For this review, use the dimensioned drawing (mm, ordinates from the lowest corner) and the shaded views. A direction names the side the tool comes from. Give positions to 0.01 mm unless a question says otherwise; leave off trailing zeros. Loops run counter-clockwise (first coordinate to the right, second up) from the corner with the lowest first, then second, coordinate; pieces in that order, holes last. Notation, with made-up numbers: M 75.25,-9.5 L 128.25,-9.5 A9 ccw 128.25,5.5 Z; hole C 84.25,37 d3. An arc over 180 degrees is marked long. Return JSON: item names as keys, results as strings.
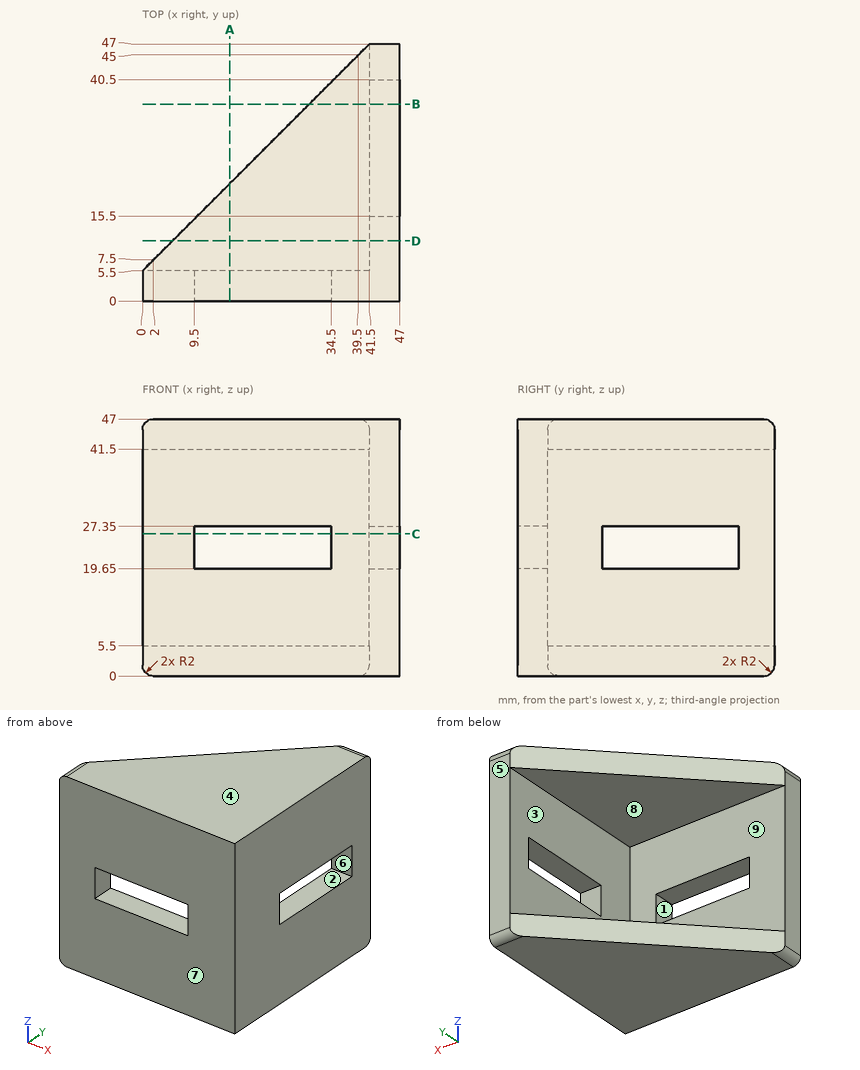
1) Tool access review of the marked faces 1, 2, 3, 4 and 5: name each direction out of +Z, -Z, +X, -X, +Y, -Y from which nothing blocks a thin tool from reaching the whole face with its end or side.
From the geometry:
{"face 1": "+Y, -Y", "face 2": "+X, -X", "face 3": "-X, +Y", "face 4": "+Z, +X, -X, +Y, -Y", "face 5": "+Z, -Z, +X, -X, +Y"}
2) Consider section A-A on x = 16. Write out the cut boundary in (y, z), then the cut area to 3 significant figures.
From the geometry:
{"outline": "M 0,0 L 21.5,0 L 21.5,5.5 L 5.5,5.5 L 5.5,19.65 L 0,19.65 Z; M 0,27.35 L 5.5,27.35 L 5.5,41.5 L 21.5,41.5 L 21.5,47 L 0,47 Z", "area": "392 mm²"}
3) Consider section C-C on z = 26. Write out the cut boundary in (x, y).
From the geometry:
{"outline": "M 0,0 L 9.5,0 L 9.5,5.5 L 0,5.5 Z; M 34.5,0 L 47,0 L 47,15.5 L 41.5,15.5 L 41.5,5.5 L 34.5,5.5 Z; M 41.5,40.5 L 47,40.5 L 47,47 L 41.5,47 Z"}
4) Consider section B-B on y = 36. Write out the cut boundary in (x, z), then the cut area to 3 significant figures.
From the geometry:
{"outline": "M 30.5,0 L 47,0 L 47,19.65 L 41.5,19.65 L 41.5,5.5 L 30.5,5.5 Z; M 30.5,41.5 L 41.5,41.5 L 41.5,27.35 L 47,27.35 L 47,47 L 30.5,47 Z", "area": "337 mm²"}
5) Wall thickness on L1, parallel to Z at x = 9.5, y = 10; L2, parallel to Y at x = 7.5, z = 15; L3, parallel to X at y = 28, z = 16: over which ranges is each line inside the solid? List them lowest first. Write a range as from..to.
From the geometry:
{"L1": "0..5.5, 41.5..47", "L2": "0..5.5", "L3": "41.5..47"}
6) The part is to be moulded in two halves that separate along Y. For the marked faces 6, 7, 8 and 9, say which applies: released by +Y, released by -Y, zero draft, split by the parting line, or undercut.
From the geometry:
{"face 6": "undercut", "face 7": "released by -Y", "face 8": "zero draft", "face 9": "released by +Y"}
7) Insertion check: pin 1 (1 mm diameter, centred on y = 33.5, z = 14, fed in from -X); pin 2 (3 mm diameter, centred on x = 26.5, z = 8, fed in from +Y); pin 3 (12 mm diameter, centred on x = 26.5, y = 41.5, fed in from -Z). Each pin has a flat end and moves straight along its axis. Give the tip position at first contact, or say it passes through.
From the geometry:
{"pin 1": "x = 41.5", "pin 2": "y = 5.5", "pin 3": "through"}
8) Consider section D-D on y = 11. Write out the cut boundary in (x, z), then the cut area to 4 significant figures.
From the geometry:
{"outline": "M 5.5,0 L 47,0 L 47,47 L 5.5,47 L 5.5,41.5 L 41.5,41.5 L 41.5,5.5 L 5.5,5.5 Z", "area": "654.5 mm²"}
